Part model, mm, in its own coordinate system. A direction names the side the tool comes from. Round coordinates to 2 decimals unless told otherwise and drop trailing zeros. Loops run counter-clockwise (first coordinate to the right, second up) from the corner with the lowest first, then second, coordinate; pieces in that order, holes last. Notation, with made-up numbers: M 86,24.25 L 117,24.25 A20 ccw 117,41.25 Z; hole C 32.25,78.5 d4. An arc over 180 degrees is marked long. Answer as CSV lines item,"result". Start each with the question number.
Item 1: Band-saw the part on B-B (x = 0). Give the cut face in (y, z), and give its area (4 significant figures).
Item 2: Mould opens along X. For faces 3 (the cylindrical face through (-11.056, -49.787, 1.479)), 4 (the flat face through (0, -5, 1)), 5 (the flat face through (-1, -11, 0)) say: pulls with the +X half, pulls with the -X half, needs draft (parallel to the pull), parting line crosses it, or undercut.
Item 3: Band-saw the part on D-D (z = 1). Give the cut face in (x, y), and give its area (3 significant figures).
Item 4: Wall check: line 1 (Y direction, x = 0, z = 2.3); line 2 (Y direction, x = -1.5, z = 0.35); line 3 (Y direction, x = -26, z = 1.75). Give the ranges that are in metal, low to high.
Item 5: Band-saw the part on C-C (y = -15). Give the cut face in (x, z), and give its area (3 significant figures).
Item 6: Drop flat-ended pins along their axis: pin 1 Ø0.9 at (x, z) = (-0.5, 1.5) entering from -Y; pin 2 Ø1.5 at (y, z) = (-15, 1.5) entering from -X; pin 3 Ø1.5 at (y, z) = (-14, 1.5) entering from +X. Give the stop position or say it passes through.
Item 7: Band-saw the part on A-A (y = 0). Give the cut face in (x, z), and give its area (3 significant figures).
Item 8: Which spindle directions (+Z, -Z, +X, -X, +Y, -Y) get a long thin tool onto all of the face, cutting with end or side? Do faces 1 (the flat face through (-1, -11, 3)), 2 (the flat face through (-5.5, -15, 1)). Say none if no direction does.
```python
from build123d import *

# Parameters (mm, degrees)
SKETCH_2_R               = 51
EXTRUDE_1_DEPTH          = 3
SKETCH_3_R               = 2.75
CUT_EXTRUDE_1_DEPTH      = 3
PATTERN_CIRCULAR_1_COUNT = 3
CUT_EXTRUDE_START        = -13.3
SKETCH_4_R               = 2.75
SKETCH_4_W               = 4
SKETCH_4_H               = 20
SKETCH_4_W_2             = 11
SKETCH_4_H_2             = 6
CUT_EXTRUDE_2_DEPTH      = 13.3


with BuildPart() as part:
    # Эскиз2 → Бобышка-Вытянуть1 (new body)
    with BuildSketch(Plane.XY):
        Circle(SKETCH_2_R)
    extrude(amount=EXTRUDE_1_DEPTH)

    # Эскиз3 → Вырез-Вытянуть1 (cut)
    with BuildSketch(Plane(origin=(0, 0, 0), x_dir=(-1, 0, 0), z_dir=(0, 0, -1))):
        with Locations((0, 30)):
            Circle(SKETCH_3_R)
    cut_extrude_1 = extrude(amount=-CUT_EXTRUDE_1_DEPTH, mode=Mode.SUBTRACT)

    # Круговой массив1: Вырез-Вытянуть1 ×3 about axis
    pattern_circular_1_axis = Axis((0, 0, 0), (0, 0, 1))
    for i in range(1, PATTERN_CIRCULAR_1_COUNT):
        add(cut_extrude_1.rotate(pattern_circular_1_axis, i * 360 / PATTERN_CIRCULAR_1_COUNT), mode=Mode.SUBTRACT)

    # Эскиз4 → Вырез-Вытянуть2 (cut)
    with BuildSketch(Plane.XY.offset(3).offset(CUT_EXTRUDE_START)):
        with Locations(Location((0, 30, 0), (0, 0, 180))):
            Circle(SKETCH_4_R)
        with Locations((0, 5)):
            Rectangle(SKETCH_4_W, SKETCH_4_H)
        with Locations((0, -15)):
            Rectangle(SKETCH_4_W_2, SKETCH_4_H_2)
    extrude(amount=CUT_EXTRUDE_2_DEPTH, mode=Mode.SUBTRACT)


solid = part.part
```
Answer block:
1,outline,"M -51,0 L -18,0 L -18,3 L -51,3 Z; M -12,0 L -5,0 L -5,3 L -12,3 Z; M 15,0 L 27.25,0 L 27.25,3 L 15,3 Z; M 32.75,0 L 51,0 L 51,3 L 32.75,3 Z"
1,area,"211.5 mm^2"
2,face 3,"parting line crosses it"
2,face 4,"undercut"
2,face 5,"needs draft"
3,outline,"C 0,0 d102; hole C -25.98,-15 d5.5; hole M -5.5,-18 L 5.5,-18 L 5.5,-12 L -5.5,-12 Z; hole C 0,30 d5.5; hole M -2,-5 L 2,-5 L 2,15 L -2,15 Z; hole C 25.98,-15 d5.5"
3,area,"7,950 mm^2"
4,line 1,"y = -51 to -18, -12 to -5, 15 to 27.25, 32.75 to 51"
4,line 2,"y = -50.98 to -18, -12 to -5, 15 to 27.7, 32.3 to 50.98"
4,line 3,"y = -43.87 to -17.75, -12.25 to 43.87"
5,outline,"M -48.74,0 L -28.73,0 L -28.73,3 L -48.74,3 Z; M -23.23,0 L -5.5,0 L -5.5,3 L -23.23,3 Z; M 5.5,0 L 23.23,0 L 23.23,3 L 5.5,3 Z; M 28.73,0 L 48.74,0 L 48.74,3 L 28.73,3 Z"
5,area,"226 mm^2"
6,pin 1,"stops at y = -51"
6,pin 2,"stops at x = -48.97"
6,pin 3,"stops at x = 49.25"
7,outline,"M -51,0 L -2,0 L -2,3 L -51,3 Z; M 2,0 L 51,0 L 51,3 L 2,3 Z"
7,area,"294 mm^2"
8,face 1,"+Z, +X, -X, +Y, -Y"
8,face 2,"+Z, -Z"
